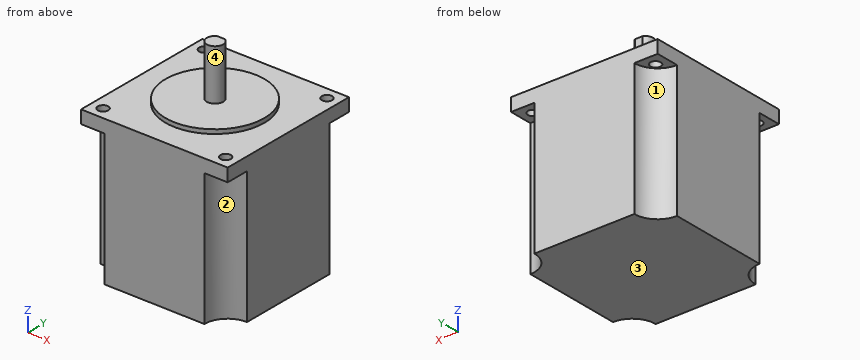
from build123d import *

# Parameters (mm, degrees)
SKETCH1_W           = 56.4
SKETCH1_H           = 56.4
BOSS_EXTRUDE1_DEPTH = 56
SKETCH2_R           = 19
BOSS_EXTRUDE2_DEPTH = 1.6
SKETCH3_R           = 3.175
BOSS_EXTRUDE3_DEPTH = 19.4
CUT_EXTRUDE1_DEPTH  = 19.4
SKETCH5_R           = 2
CUT_EXTRUDE2_DEPTH  = 69.749399997
SKETCH6_R           = 9
CUT_EXTRUDE3_DEPTH  = 51


with BuildPart() as part:
    # Sketch1 → Boss-Extrude1 (new body)
    with BuildSketch(Plane.XY):
        Rectangle(SKETCH1_W, SKETCH1_H)
    extrude(amount=BOSS_EXTRUDE1_DEPTH)

    # Sketch2 → Boss-Extrude2 (add)
    with BuildSketch(Plane.XY.offset(56)):
        Circle(SKETCH2_R)
    extrude(amount=BOSS_EXTRUDE2_DEPTH)

    # Sketch3 → Boss-Extrude3 (add)
    with BuildSketch(Plane.XY.offset(57.6)):
        Circle(SKETCH3_R)
    extrude(amount=BOSS_EXTRUDE3_DEPTH)

    # Sketch4 → Cut-Extrude1 (cut)
    with BuildSketch(Plane.XY.offset(77)):
        Polygon((-97.277384537, 2.825), (-1.449137675, 2.825), (1.449137675, 2.825), (97.277384537, 2.825), (97.277384537, 194.481493724), (-97.277384537, 194.481493724), align=None)
    extrude(amount=-CUT_EXTRUDE1_DEPTH, mode=Mode.SUBTRACT)

    # Sketch5 → Cut-Extrude2 (cut, through all)
    with BuildSketch(Plane.XY.offset(56)):
        with Locations((23.57, 23.57)):
            Circle(SKETCH5_R)
        with Locations(Location((-23.57, 23.57, 0), (0, 0, 180))):
            Circle(SKETCH5_R)
        with Locations(Location((23.57, -23.57, 0), (0, 0, 180))):
            Circle(SKETCH5_R)
        with Locations((-23.57, -23.57)):
            Circle(SKETCH5_R)
    extrude(amount=-CUT_EXTRUDE2_DEPTH, mode=Mode.SUBTRACT)

    # Sketch6 → Cut-Extrude3 (cut)
    with BuildSketch(Plane(origin=(0, 0, 0), x_dir=(-1, 0, 0), z_dir=(0, 0, -1))):
        with Locations((-28.2, 28.2)):
            Circle(SKETCH6_R)
        with Locations((-28.2, -28.2)):
            Circle(SKETCH6_R)
        with Locations((28.2, -28.2)):
            Circle(SKETCH6_R)
        with Locations((28.2, 28.2)):
            Circle(SKETCH6_R)
    extrude(amount=-CUT_EXTRUDE3_DEPTH, mode=Mode.SUBTRACT)


solid = part.part
The listing builds one solid part. Answer for the finished solid, in the listing's coordinates (mm). Face numbers are marked on the shaded views. A direction names the side the tool comes from. Coordinates: 2 decimals unless noted, no trailing zeros. Loops run counter-clockwise (first coordinate to the right, second up) from the corner with the lowest first, then second, coordinate; pieces in that order, holes last.
1) Flat-ended cylindrical pins translate along their axes: pin 1 Ø2.5 at (x, z) = (0, 66) entering from +Y (3 decimals); pin 2 Ø8 at (x, y) = (-11.5, 4.5) entering from +Z; pin 3 Ø2.5 at (x, y) = (-24.5, -24.5) entering from -Z. Find the tip coordinate at first contact, or state that the pin passes through.
2) Find section D-D on y = -23.57. Write down the section's boundary in (x, z).
3) Find section C-C on y = 0. Write down the section's boundary in (x, z) (3 decimals).
4) Find section A-A on z = 31. Write down the section's boundary in (x, y), then the cut area to 3 significant figures.
5) Find the intervals of material crossed by L1, parallel to Y at x = 23.57, z = 55.05; L2, parallel to Z at x = -4, y = 20.5, in increasing order.
6) A tool of negligible diameter and unlimited length cuts with its end or side. For the marked faces 1, 2, 3 and 4, from which of +Z, -Z, +X, -X, +Y, -Y can it reach the whole face along a straight path? Write none if from no direction.
7) Find section B-B on x = 0. Write down the section's boundary in (y, z) (3 decimals).
Values:
1. pin 1: stops at y = 2.825
1. pin 2: stops at z = 57.6
1. pin 3: stops at z = 51
2. outline: (-28.2, 51) - (-25.57, 51) - (-25.57, 56) - (-28.2, 56) - close; (-21.57, 51) - (-20.48, 51) - (-20.48, 0) - (20.48, 0) - (20.48, 51) - (21.57, 51) - (21.57, 56) - (-21.57, 56) - close; (25.57, 51) - (28.2, 51) - (28.2, 56) - (25.57, 56) - close
3. outline: (-28.2, 0) - (28.2, 0) - (28.2, 56) - (19, 56) - (19, 57.6) - (3.175, 57.6) - (3.175, 77) - (-3.175, 77) - (-3.175, 57.6) - (-19, 57.6) - (-19, 56) - (-28.2, 56) - close
4. outline: (-28.2, -19.2) arc R9 cw to (-19.2, -28.2) - (19.2, -28.2) arc R9 cw to (28.2, -19.2) - (28.2, 19.2) arc R9 cw to (19.2, 28.2) - (-19.2, 28.2) arc R9 cw to (-28.2, 19.2) - close
4. area: 2,930 mm2
5. L1: y = -28.2 to -25.57, -21.57 to 21.57, 25.57 to 28.2
5. L2: z = 0 to 56
6. face 1: -Z, -X, +Y
6. face 2: -Z, +X, -Y
6. face 3: -Z, +X, -X, +Y, -Y
6. face 4: +Z
7. outline: (-28.2, 0) - (28.2, 0) - (28.2, 56) - (19, 56) - (19, 57.6) - (2.825, 57.6) - (2.825, 77) - (-3.175, 77) - (-3.175, 57.6) - (-19, 57.6) - (-19, 56) - (-28.2, 56) - close
